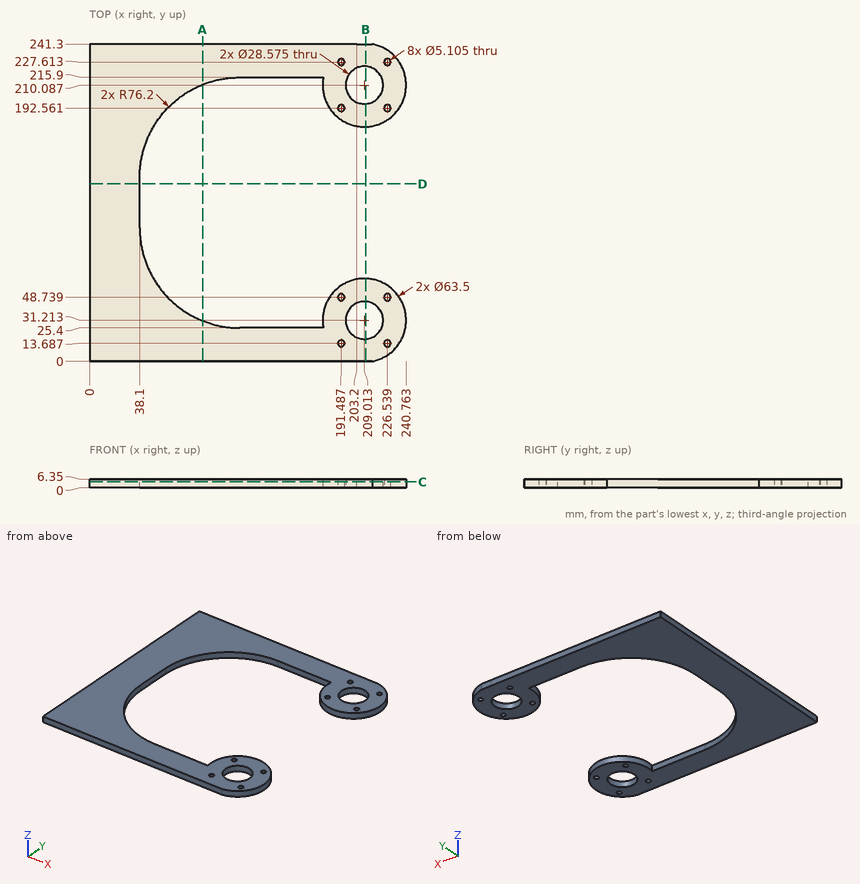
Can you work these out from the drawing? Everything is in mm from the part's minimum corner. Round coordinates to 2 decimals unless told otherwise and drop trailing zeros. Write each loop counter-clockwise with the first axis right and the second up, starting at its lowest first coordinate (ties: lowest second). Pieces come first, ordered by that corner, then holes. Notation, with made-up numbers: M 77,12 L 122,12 A20 cw 122,41 Z; hole C 77,-10 d7. An arc over 180 degrees is marked long. Use a Markdown table: item, result.
Item 1: If I drill on line 1 along Y through (x, z) = (173, 1); line 2 along X through (y, z) = (204.5, 1.5) (1 decimal); line 3 along Y through (x, z) = (210.5, 5.5), over which ranges is the centre line in solid material (lowest first)? Write a range as [from, to].
Found:
| item | result |
|---|---|
| line 1 | y = [0, 25.4], [215.9, 241.3] |
| line 2 | x = [0, 74.2], [177.8, 195.9], [222.2, 240.3] |
| line 3 | y = [0, 17], [45.42, 62.93], [178.37, 195.88], [224.3, 241.3] |
Item 2: I want a section at A-A (x = 86). List the corners of the cut face in (y, z) for me, and give its area (3 significant figures).
Found:
| item | result |
|---|---|
| outline | M 0,0 L 30.85,0 L 30.85,6.35 L 0,6.35 Z; M 210.45,0 L 241.3,0 L 241.3,6.35 L 210.45,6.35 Z |
| area | 392 mm2 |
Item 3: I want a section at B-B (x = 210). List the corners of the cut face in (y, z) for me.
Found:
| item | result |
|---|---|
| outline | M 0,0 L 16.96,0 L 16.96,6.35 L 0,6.35 Z; M 45.47,0 L 62.95,0 L 62.95,6.35 L 45.47,6.35 Z; M 178.35,0 L 195.83,0 L 195.83,6.35 L 178.35,6.35 Z; M 224.34,0 L 241.3,0 L 241.3,6.35 L 224.34,6.35 Z |
Item 4: I want a section at C-C (z = 4.5). State how many separate pieces and enclosed holes the cut face has, and give its area (3 significant figures).
Found:
| item | result |
|---|---|
| separate pieces | 1 |
| enclosed holes | 10 |
| area | 24,000 mm2 |
Item 5: I want a section at D-D (y = 135). List the corners of the cut face in (x, z) for me.
Found:
| item | result |
|---|---|
| outline | M 0,0 L 38.1,0 L 38.1,6.35 L 0,6.35 Z |
Item 6: For pin 1 Ø1.9 at (y, z) = (115.5, 1.5) entering from +X, with a flat end and sliding along its axis, tell me the tip position at first contact or that it passes through.
Found:
| item | result |
|---|---|
| pin 1 | stops at x = 38.1 |
